Could you check a few things on this model? Use its own coordinates, in mm. Face numbers are marked on the shaded views. A direction names the side the tool comes from. Coordinates: 2 decimals unless noted, no trailing zeros. Order: outer loops, then holes, each group sorted by start corner. A loop starts at its lowest first (then second) coordinate and runs counter-clockwise, first axis right, second up. Notation, with made-up numbers: (-39, 3.25) - (17, 3.25) arc R21 ccw to (17, 11.25) - close; hole circle Ø10 at (-35, -10.5). An arc over 180 degrees is marked (long way). One line per item, written item: value.
from build123d import *

# Parameters (mm, degrees)
BASE_FLANGE2_DEPTH         = 475
SKETCH13_R                 = 2.25
CUT_EXTRUDE4_DEPTH         = 700.483927325
SKETCH14_R                 = 11.5
SKETCH14_R_2               = 1.75
STEPPER_MOTOR_CUTOUT_DEPTH = 0.889
SKETCH15_R                 = 2.25
CUT_EXTRUDE6_DEPTH         = 0.889
SKETCH16_W                 = 46.8
SKETCH16_H                 = 27
CUT_EXTRUDE7_DEPTH         = 0.889
M4_CLEARANCE_HOLE1_D       = 4.5


# Sheet-metal steps are written as plain solids
with BuildPart() as part:
    # Sketch1 → Base-Flange2 (new body)
    with BuildSketch(Plane(origin=(0, 0, 0), x_dir=(1, 0, 0), z_dir=(0, 1, 0))):
        with BuildLine():
            Line((195.849919955, 332), (195.849919955, 12.7))
            ThreePointArc((195.849919955, 12.7), (192.130176076, 3.719743879), (183.149919955, 0))
            Line((183.149919955, 0), (-183.149919955, 0))
            ThreePointArc((-183.149919955, 0), (-192.130176076, 3.719743879), (-195.849919955, 12.7))
            Line((-195.849919955, 12.7), (-195.849919955, 332))
            Line((-195.849919955, 332), (-194.960919955, 332))
            Line((-194.960919955, 332), (-194.960919955, 12.7))
            ThreePointArc((-194.960919955, 12.7), (-191.501558148, 4.348361807), (-183.149919955, 0.889))
            Line((-183.149919955, 0.889), (183.149919955, 0.889))
            ThreePointArc((183.149919955, 0.889), (191.501558148, 4.348361807), (194.960919955, 12.7))
            Line((194.960919955, 12.7), (194.960919955, 332))
            Line((194.960919955, 332), (195.849919955, 332))
        make_face()
    extrude(amount=BASE_FLANGE2_DEPTH)

    # Sketch13 → Cut-Extrude4 (cut, through all)
    with BuildSketch(Plane(origin=(195.849919955, 0, 0), x_dir=(0, 0, -1), z_dir=(1, 0, 0))):
        with Locations((50.096107, 60)):
            Circle(SKETCH13_R)
        with Locations((50.096107, 316.132840032)):
            Circle(SKETCH13_R)
        with Locations((50.096107, 30)):
            Circle(SKETCH13_R)
    extrude(amount=-CUT_EXTRUDE4_DEPTH, mode=Mode.SUBTRACT)

    # Sketch14 → Stepper motor cutout (cut)
    with BuildSketch(Plane.XY):
        with Locations((49.936500045, 311.73292)):
            Circle(SKETCH14_R)
        with Locations((34.436500045, 296.23292)):
            Circle(SKETCH14_R_2)
        with Locations((65.436500045, 296.23292)):
            Circle(SKETCH14_R_2)
        with Locations((34.436500045, 327.23292)):
            Circle(SKETCH14_R_2)
        with Locations((65.436500045, 327.23292)):
            Circle(SKETCH14_R_2)
        with Locations((80.936500045, 255.73292)):
            Circle(SKETCH14_R)
        with Locations((65.436500045, 240.23292)):
            Circle(SKETCH14_R_2)
        with Locations((96.436500045, 240.23292)):
            Circle(SKETCH14_R_2)
        with Locations((65.436500045, 271.23292)):
            Circle(SKETCH14_R_2)
        with Locations((96.436500045, 271.23292)):
            Circle(SKETCH14_R_2)
    extrude(amount=-STEPPER_MOTOR_CUTOUT_DEPTH, mode=Mode.SUBTRACT)

    # Sketch15 → Cut-Extrude6 (cut)
    with BuildSketch(Plane.XY):
        with Locations((-145.753812955, 316.132839976)):
            Circle(SKETCH15_R)
        with Locations((-118.946026845, 316.132839976)):
            Circle(SKETCH15_R)
        with Locations((118.946026845, 316.132839976)):
            Circle(SKETCH15_R)
        with Locations((145.753812955, 316.132839976)):
            Circle(SKETCH15_R)
        with Locations((145.753812955, 30)):
            Circle(SKETCH15_R)
        with Locations((118.946026845, 30)):
            Circle(SKETCH15_R)
        with Locations((-118.946026845, 30)):
            Circle(SKETCH15_R)
        with Locations((-145.753812955, 30)):
            Circle(SKETCH15_R)
    extrude(amount=-CUT_EXTRUDE6_DEPTH, mode=Mode.SUBTRACT)

    # Sketch16 → Cut-Extrude7 (cut)
    with BuildSketch(Plane.XY):
        with Locations((-73.4, 23.5)):
            Rectangle(SKETCH16_W, SKETCH16_H)
    extrude(amount=-CUT_EXTRUDE7_DEPTH, mode=Mode.SUBTRACT)

    # M4 Clearance Hole1 (through all)
    with Locations(Plane.XY):
        with Locations((-75.063499955, 181.73292), (-75.063499955, 171.73292)):
            Hole(M4_CLEARANCE_HOLE1_D / 2)


solid = part.part
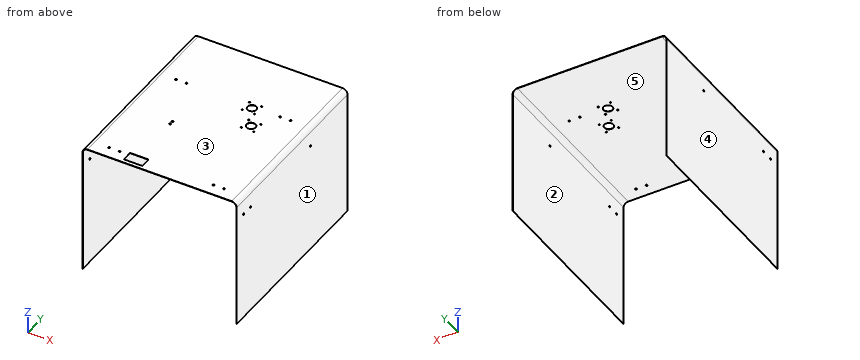
Item 1: I want a section at C-C on x = -31. Please give me the cut outline in (y, z), then the cut area to 3 significant figures.
Conclusion:
outline: (0, -0.89) - (475, -0.89) - (475, 0) - (0, 0) - close
area: 422 mm²
Item 2: If I drill on probe 1 along X at (y, z) = (166.5, -143.5); probe 2 along Z at (x, y) = (-172.5, 285.5), over which ranges is the centre line in solid material (lowest first)?
Conclusion:
probe 1: -195.85 to -194.96, 194.96 to 195.85
probe 2: -0.89 to 0
Item 3: I'm going to push flat-ended pins straight in: pin 1 Ø4 at (y, z) = (30, -50.1) entering from -X; pin 2 Ø12 at (x, y) = (-123.5, 173.5) entering from -Z. Where does each tip first touch, or does it pass through?
Conclusion:
pin 1: through
pin 2: z = -0.89
Item 4: I want a section at A-A on z = -280.5. Please give me the cut outline in (x, y).
Conclusion:
outline: (-195.85, 0) - (-194.96, 0) - (-194.96, 475) - (-195.85, 475) - close; (194.96, 0) - (195.85, 0) - (195.85, 475) - (194.96, 475) - close
Item 5: I want a section at B-B on y = 232. Please give me the cut outline in (x, z), then the cut area to 3 significant figures.
Conclusion:
outline: (-195.85, -332) - (-194.96, -332) - (-194.96, -12.7) arc R11.81 cw to (-183.15, -0.89) - (183.15, -0.89) arc R11.81 cw to (194.96, -12.7) - (194.96, -332) - (195.85, -332) - (195.85, -12.7) arc R12.7 ccw to (183.15, 0) - (-183.15, 0) arc R12.7 ccw to (-195.85, -12.7) - close
area: 928 mm²
Item 6: Thinking about a two-plate mould opening in X: for the marked faces 1, 2 and 3, which applies, pulls with the +X half, pulls with the -X half, needs draft (parallel to the pull), parting line crosses it, or undercut?
Conclusion:
face 1: pulls with the +X half
face 2: undercut
face 3: needs draft
Item 7: For the marked faces 4 and 5, which set-ups out of +Z, -Z, +X, -X, +Y, -Y let a thin tool reach every point of the face, with its end or its side?
Conclusion:
face 4: +Z, -Z, -X, +Y, -Y
face 5: -Z, +Y, -Y
